```python
from build123d import *

# Parameters (mm, degrees)
BOSS_EXTRUDE1_DEPTH             = 30
SKETCH2_R                       = 1.75
CUT_EXTRUDE1_DEPTH              = 8
SKETCH5_R                       = 1.75
CUT_EXTRUDE2_DEPTH              = 3
BOSS_EXTRUDE2_DEPTH             = 3
CIRPATTERN5_COUNT               = 4
SKETCH4_W                       = 48
SKETCH4_H                       = 48
SKETCH4_W_2                     = 42
SKETCH4_H_2                     = 42
BOSS_EXTRUDE3_DEPTH             = 115
SKETCH6_W                       = 48
SKETCH6_H                       = 48
BOSS_EXTRUDE4_DEPTH             = 4
SKETCH7_R                       = 2
CUT_EXTRUDE3_DEPTH              = 4
CUT_EXTRUDE4_DEPTH              = 163.262133599
BOSS_EXTRUDE5_REACH             = 164.262
BOSS_EXTRUDE5_DIRECTION_2_REACH = 164.262
CIRPATTERN6_COUNT               = 4


with BuildPart() as part:
    # Sketch1 → Boss-Extrude1 (new body)
    with BuildSketch(Plane(origin=(0, 0, 0), x_dir=(1, 0, 0), z_dir=(0, 1, 0))):
        Polygon((48.25, -78), (48.25, -50.371320344), (20.152543264, -22.273863607), (21.213203436, -21.213203436), (50.75, -50.75), (50.75, -70), (64.007359313, -70), (67.003679656, -67.003679656), (69.125, -69.125), (60.25, -78), align=None)
    boss_extrude1 = extrude(amount=BOSS_EXTRUDE1_DEPTH)

    # Sketch2 → Cut-Extrude1 (cut)
    with BuildSketch(Plane.XY.offset(78)):
        with Locations((54.25, 5)):
            Circle(SKETCH2_R)
        with Locations((54.25, 25)):
            Circle(SKETCH2_R)
    cut_extrude1 = extrude(amount=-CUT_EXTRUDE1_DEPTH, mode=Mode.SUBTRACT)

    # Mirror1: Boss-Extrude1, Cut-Extrude1 across plane
    add(boss_extrude1.mirror(Plane(origin=(50.75, 30, 50.75), x_dir=(0.707106781186549, 0, 0.707106781186546), z_dir=(-0.707106781186546, 0, 0.707106781186549))))
    add(cut_extrude1.mirror(Plane(origin=(50.75, 30, 50.75), x_dir=(0.707106781186549, 0, 0.707106781186546), z_dir=(-0.707106781186546, 0, 0.707106781186549))), mode=Mode.SUBTRACT)

    # Sketch5 → Cut-Extrude2 (cut)
    with BuildSketch(Plane(origin=(69.125, 0, 69.125), x_dir=(0.7071067811865461, 0, -0.7071067811865489), z_dir=(0.7071067811865489, 0, 0.7071067811865461))):
        with Locations((0, 25)):
            Circle(SKETCH5_R)
        with Locations((0, 5)):
            Circle(SKETCH5_R)
    extrude(amount=-CUT_EXTRUDE2_DEPTH, mode=Mode.SUBTRACT)

    # Sketch3 → Boss-Extrude2 (add)
    with BuildSketch(Plane(origin=(-1.060660172, 0, 1.060660172), x_dir=(0.7071067811865492, 0, 0.7071067811865459), z_dir=(-0.7071067811865459, 0, 0.7071067811865492))):
        Polygon((30, 30), (30, 65), (68, 30), align=None)
    extrude(amount=-BOSS_EXTRUDE2_DEPTH)


with BuildPart() as cirpattern5_1:
    # CirPattern5: pattern copy
    add(part.part.rotate(Axis((0, 0, 0), (0, 1, 0)), 1 * 360 / CIRPATTERN5_COUNT))


with BuildPart() as cirpattern5_2:
    # CirPattern5: pattern copy
    add(part.part.rotate(Axis((0, 0, 0), (0, 1, 0)), 2 * 360 / CIRPATTERN5_COUNT))


with BuildPart() as cirpattern5_3:
    # CirPattern5: pattern copy
    add(part.part.rotate(Axis((0, 0, 0), (0, 1, 0)), 3 * 360 / CIRPATTERN5_COUNT))


with BuildPart() as part_1:
    add(part.part)

    add(cirpattern5_1.part)  # Boss-Extrude3 merges CirPattern5_1

    add(cirpattern5_2.part)  # Boss-Extrude3 merges CirPattern5_2

    add(cirpattern5_3.part)  # Boss-Extrude3 merges CirPattern5_3
    # Sketch4 → Boss-Extrude3 (add)
    with BuildSketch(Plane.XZ):
        Rectangle(SKETCH4_W, SKETCH4_H)
        Rectangle(SKETCH4_W_2, SKETCH4_H_2, mode=Mode.SUBTRACT)
    extrude(amount=-BOSS_EXTRUDE3_DEPTH)

    # Sketch6 → Boss-Extrude4 (add)
    with BuildSketch(Plane(origin=(0, 115, 0), x_dir=(1, 0, 0), z_dir=(0, 1, 0))):
        Rectangle(SKETCH6_W, SKETCH6_H)
    extrude(amount=BOSS_EXTRUDE4_DEPTH)

    # Sketch7 → Cut-Extrude3 (cut)
    with BuildSketch(Plane(origin=(0, 119, 0), x_dir=(1, 0, 0), z_dir=(0, 1, 0))):
        with Locations(Location((16, 16, 0), (0, 0, 270))):
            Circle(SKETCH7_R)
        with Locations(Location((-16, 16, 0), (0, 0, 270))):
            Circle(SKETCH7_R)
        with Locations(Location((-16, -16, 0), (0, 0, 270))):
            Circle(SKETCH7_R)
        with Locations(Location((16, -16, 0), (0, 0, 270))):
            Circle(SKETCH7_R)
    extrude(amount=-CUT_EXTRUDE3_DEPTH, mode=Mode.SUBTRACT)

    # Sketch8 → Cut-Extrude4 (cut, symmetric)
    with BuildSketch(Plane(origin=(0, 0, 0), x_dir=(0.7071067811865475, 0, -0.7071067811865477), z_dir=(0.7071067811865477, 0, 0.7071067811865475))):
        with BuildLine():
            Line((-33.941125497, 87.751594937), (-33.941125497, 62.751594937))
            ThreePointArc((-33.941125497, 62.751594937), (-26.941125497, 75.251594937), (-33.941125497, 87.751594937))
        make_face()
    cut_extrude4 = extrude(amount=CUT_EXTRUDE4_DEPTH, both=True, mode=Mode.SUBTRACT)

    # Sketch9 → Boss-Extrude5 (add, up to next)
    with BuildSketch(Plane(origin=(0, 0, 0), x_dir=(0.7071067811865475, 0, -0.7071067811865477), z_dir=(0.7071067811865477, 0, 0.7071067811865475)), mode=Mode.PRIVATE) as boss_extrude5_sk1:
        with BuildLine():
            Line((-29.69848481, 83.810022582), (-29.69848481, 88.298087549))
            ThreePointArc((-29.69848481, 88.298087549), (-23.941125497, 75.251594937), (-29.69848481, 62.205102325))
            Line((-29.69848481, 62.205102325), (-29.69848481, 66.693167292))
            ThreePointArc((-29.69848481, 66.693167292), (-26.941125497, 75.251594937), (-29.69848481, 83.810022582))
        make_face()
    boss_extrude5_tool1 = extrude(boss_extrude5_sk1.sketch, amount=BOSS_EXTRUDE5_REACH, mode=Mode.PRIVATE) - part_1.part
    boss_extrude5 = boss_extrude5_tool1.solids().sort_by_distance((-18.95893, 75.251595, 18.95893))[0]
    add(boss_extrude5)

    # Sketch9 → Boss-Extrude5 direction 2 (add, up to next)
    with BuildSketch(Plane(origin=(0, 0, 0), x_dir=(0.7071067811865475, 0, -0.7071067811865477), z_dir=(0.7071067811865477, 0, 0.7071067811865475)), mode=Mode.PRIVATE) as boss_extrude5_direction_2_sk1:
        with BuildLine():
            Line((-29.69848481, 83.810022582), (-29.69848481, 88.298087549))
            ThreePointArc((-29.69848481, 88.298087549), (-23.941125497, 75.251594937), (-29.69848481, 62.205102325))
            Line((-29.69848481, 62.205102325), (-29.69848481, 66.693167292))
            ThreePointArc((-29.69848481, 66.693167292), (-26.941125497, 75.251594937), (-29.69848481, 83.810022582))
        make_face()
    boss_extrude5_direction_2_tool1 = extrude(boss_extrude5_direction_2_sk1.sketch, amount=-BOSS_EXTRUDE5_DIRECTION_2_REACH, mode=Mode.PRIVATE) - part_1.part
    boss_extrude5_direction_2 = boss_extrude5_direction_2_tool1.solids().sort_by_distance((-18.95893, 75.251595, 18.95893))[0]
    add(boss_extrude5_direction_2)

    # CirPattern6: Cut-Extrude4, Boss-Extrude5, Boss-Extrude5 direction 2 ×4 about axis
    cirpattern6_axis = Axis((0, 31.5, 0), (0, -1, 0))
    add([cut_extrude4.rotate(cirpattern6_axis, i * 360 / CIRPATTERN6_COUNT) for i in range(1, CIRPATTERN6_COUNT)], mode=Mode.SUBTRACT)
    add([boss_extrude5.rotate(cirpattern6_axis, i * 360 / CIRPATTERN6_COUNT) for i in range(1, CIRPATTERN6_COUNT)])
    add([boss_extrude5_direction_2.rotate(cirpattern6_axis, i * 360 / CIRPATTERN6_COUNT) for i in range(1, CIRPATTERN6_COUNT)])


solid = part_1.part
```
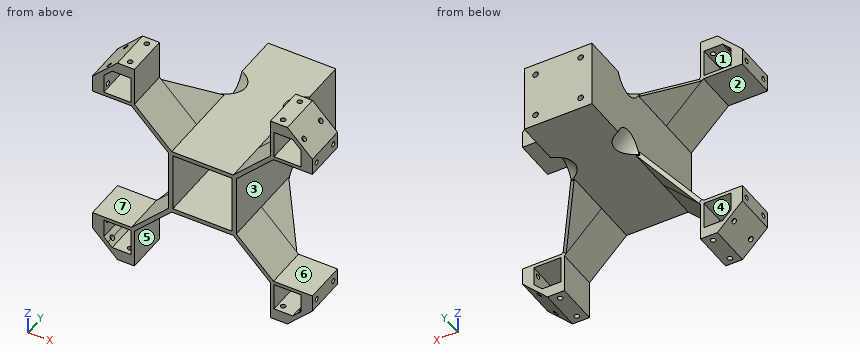
The listing builds one solid part. Answer for the finished solid, in the listing's coordinates (mm). Face numbers are marked on the shaded views. A direction names the side the tool comes from. Coordinates: 2 decimals unless noted, no trailing zeros. Loops run counter-clockwise (first coordinate to the right, second up) from the corner with the lowest first, then second, coordinate; pieces in that order, holes last. Notation, with made-up numbers: (62, 18.5) -> (68, 18.5) arc R26 ccw to (68, 32.5) -> close; hole circle Ø7 at (85.5, 25). An arc over 180 degrees is marked (long way). Use one line per item in the form item = value. Start each with the question number.
Item 1: A tool of negligible diameter and unlimited length cuts with its end or side. For the marked faces 4, 5, 6 and 7, from which of +Z, -Z, +X, -X, +Y, -Y can it reach the whole face along a straight path? Write none if from no direction.
Item 2: The part is cut by section C-C on y = 34. Determine the outline of the cut face in (x, z).
Item 3: The part is cut by section B-B on z = -30. Determine the outline of the cut face in (x, y).
Item 4: The part is cut by section A-A on y = 100. Determine the outline of the cut face in (x, z).
Item 5: Consider L1, parallel to Y at x = -72.25, z = 54.25; L2, parallel to X at y = 21, z = 63.5; L3, parallel to X at y = 80.5, z = 0.5. Determine where each line is inside the solid, lowest interval first. Write a range as [from, to].
Item 6: Flat-ended cylindrical pins translate along their axes: pin 1 Ø14.5 at (x, y) = (-3, 80) entering from +Z; pin 2 Ø3 at (y, z) = (25, -54.25) entering from +X; pin 3 Ø6 at (x, y) = (-64.5, 9.5) entering from -Z; pin 4 Ø8 at (x, y) = (42, 47.5) entering from +Z. Find the tip coordinate at first contact, or state that the pin passes through.
Item 7: The part is cut by section D-D on y = 67.5. Determine the outline of the cut face in (x, z).
Item 8: The mould has two halves that part along X. Classify the marked faces 1, 2 and 3: released by +X, released by -X, zero draft, split by the parting line, or undercut.
Answer key:
q1.face_4 = +Y, -Y
q1.face_5 = -Z, +Y, -Y
q1.face_6 = +X, +Y, -Y
q1.face_7 = -X, +Y, -Y
q2.outline = (-46.07, -43.95) -> (-43.95, -46.07) -> (-21.88, -24) -> (21.88, -24) -> (43.95, -46.07) -> (46.07, -43.95) -> (24, -21.88) -> (24, 21.88) -> (46.07, 43.95) -> (43.95, 46.07) -> (21.88, 24) -> (-21.88, 24) -> (-43.95, 46.07) -> (-46.07, 43.95) -> (-24, 21.88) -> (-24, -21.88) -> close; hole (-21, -21) -> (21, -21) -> (21, 21) -> (-21, 21) -> close
q3.outline = (-32.12, 0) -> (-27.88, 0) -> (-27.88, 54.94) -> (-32.12, 52.17) -> close; (27.88, 0) -> (32.12, 0) -> (32.12, 52.17) -> (27.88, 54.94) -> close
q4.outline = (-24, -24) -> (24, -24) -> (24, 24) -> (-24, 24) -> close; hole (-21, -21) -> (21, -21) -> (21, 21) -> (-21, 21) -> close
q5.L1 = [0, 3.25], [6.75, 23.25], [26.75, 30]
q5.L2 = [-74.75, -70], [-50.75, -48.25], [48.25, 50.75], [70, 74.75]
q5.L3 = [-24, -21], [21, 24]
q6.pin_1 = 24
q6.pin_2 = 50.75
q6.pin_3 = -76.75
q6.pin_4 = through
q7.outline = (-24, -17.24) -> (-17.24, -24) -> (17.24, -24) -> (24, -17.24) -> (24, 17.24) -> (17.24, 24) -> (-17.24, 24) -> (-24, 17.24) -> close; hole (-21, -15.39) -> (-15.39, -21) -> (15.39, -21) -> (21, -15.39) -> (21, 15.39) -> (15.39, 21) -> (-15.39, 21) -> (-21, 15.39) -> close
q8.face_1 = undercut
q8.face_2 = zero draft
q8.face_3 = released by +X
